Source: CAD feature listing. Evaluate the final solid. Frame: model axes, mm. Face numbers are marked on the shaded views. A direction names the side the tool comes from. Round coordinates to 2 decimals unless told otherwise and drop trailing zeros. Write each loop counter-clockwise with the first axis right and the second up, starting at its lowest first coordinate (ties: lowest second). Pieces come first, ordered by that corner, then holes. Notation, with made-up numbers: M 23.25,-2.75 L 44.25,-2.75 A12 cw 44.25,16.25 Z; hole C -5.75,-11.5 d6. An arc over 180 degrees is marked long. Answer in a Markdown table with one row per item.
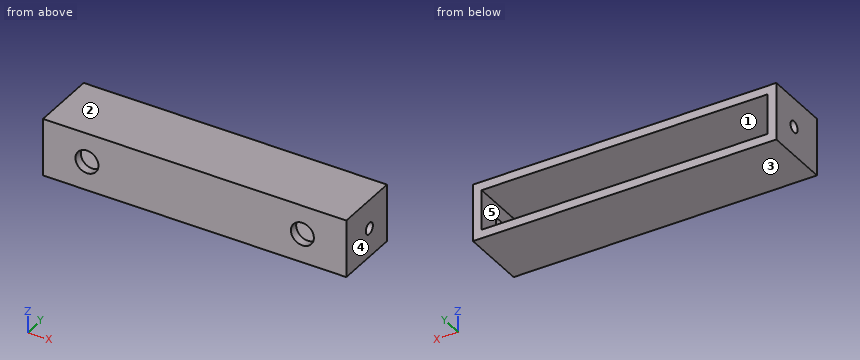
from build123d import *

# Parameters (mm, degrees)
SKETCH_1_W          = 105.6
SKETCH_1_H          = 20
SKETCH_1_R          = 4
EXTRUDE_1_DEPTH     = 3
SKETCH_10_W         = 105.6
SKETCH_10_H         = 20
SKETCH_10_W_2       = 99.6
SKETCH_10_H_2       = 14
EXTRUDE_2_DEPTH     = 20
SKETCH_11_R         = 2
CUT_EXTRUDE_1_DEPTH = 110


with BuildPart() as part:
    # 草图1 → 凸台-拉伸1 (new body)
    with BuildSketch(Plane(origin=(0, 0, 0), x_dir=(1, 0, 0), z_dir=(0, 1, 0))):
        Rectangle(SKETCH_1_W, SKETCH_1_H)
        with Locations((-37.5, 0)):
            Circle(SKETCH_1_R, mode=Mode.SUBTRACT)
        with Locations((37.5, 0)):
            Circle(SKETCH_1_R, mode=Mode.SUBTRACT)
    extrude(amount=EXTRUDE_1_DEPTH)

    # 草图10 → 凸台-拉伸2 (add)
    with BuildSketch(Plane(origin=(0, 3, 0), x_dir=(1, 0, 0), z_dir=(0, 1, 0))):
        Rectangle(SKETCH_10_W, SKETCH_10_H)
        Rectangle(SKETCH_10_W_2, SKETCH_10_H_2, mode=Mode.SUBTRACT)
    extrude(amount=EXTRUDE_2_DEPTH)

    # 草图11 → 切除-拉伸1 (cut)
    with BuildSketch(Plane.ZY.offset(52.8)):
        with Locations((0, 13)):
            Circle(SKETCH_11_R)
    extrude(amount=-CUT_EXTRUDE_1_DEPTH, mode=Mode.SUBTRACT)


solid = part.part
Q1. Section A-A (x = 37.5). Return loops of the section in (y, z), and give its area (3 significant figures).
Solutions:
| item | result |
|---|---|
| outline | M 0,-10 L 23,-10 L 23,-7 L 3,-7 L 3,-4 L 0,-4 Z; M 0,4 L 3,4 L 3,7 L 23,7 L 23,10 L 0,10 Z |
| area | 156 mm2 |
Q2. Contact query for flat-ended pins moving along their axis: pin 1 Ø9 at (x, z) = (37.5, 0) entering from +Y; pin 2 Ø5 at (x, z) = (-37.5, 0) entering from -Y. Output: stop coordinate, or through.
Solutions:
| item | result |
|---|---|
| pin 1 | stops at y = 3 |
| pin 2 | passes through |
Q3. Access query for the marked faces 1 and 2. Directions: +Z, -Z, +X, -X, +Y, -Y. A direction counts if a zero-diameter tool reaches every point of the face in a straight line with its end or side. Return the directions, or none.
Solutions:
| item | result |
|---|---|
| face 1 | +Y |
| face 2 | +Z, +X, -X, +Y, -Y |
Q4. Section D-D (x = -18). Return loops of the section in (y, z), and give its area (3 significant figures).
Solutions:
| item | result |
|---|---|
| outline | M 0,-10 L 23,-10 L 23,-7 L 3,-7 L 3,7 L 23,7 L 23,10 L 0,10 Z |
| area | 180 mm2 |
Q5. Section B-B (z = 0). Return loops of the section in (x, y), and give its area (3 significant figures).
Solutions:
| item | result |
|---|---|
| outline | M -52.8,0 L -41.5,0 L -41.5,3 L -49.8,3 L -49.8,11 L -52.8,11 Z; M -52.8,15 L -49.8,15 L -49.8,23 L -52.8,23 Z; M -33.5,0 L 33.5,0 L 33.5,3 L -33.5,3 Z; M 41.5,0 L 52.8,0 L 52.8,11 L 49.8,11 L 49.8,3 L 41.5,3 Z; M 49.8,15 L 52.8,15 L 52.8,23 L 49.8,23 Z |
| area | 365 mm2 |
Q6. Pull-direction query (Z, two-part tool) for the marked faces 3, 4 and 5; classes: pulls with the +Z half, pulls with the -Z half, needs draft (parallel to the pull), parting line crosses it, or undercut.
Solutions:
| item | result |
|---|---|
| face 3 | pulls with the -Z half |
| face 4 | needs draft |
| face 5 | undercut |
Q7. Section C-C (y = 13). Return loops of the section in (x, z).
Solutions:
| item | result |
|---|---|
| outline | M -52.8,-10 L 52.8,-10 L 52.8,-2 L 49.8,-2 L 49.8,-7 L -49.8,-7 L -49.8,-2 L -52.8,-2 Z; M -52.8,2 L -49.8,2 L -49.8,7 L 49.8,7 L 49.8,2 L 52.8,2 L 52.8,10 L -52.8,10 Z |
Q8. Material intervals for probe 1 along X at (y, z) = (1.85, 0); probe 2 along Z at (x, y) = (-24, 12); probe 3 along Z at (x, y) = (37.5, 2), sorted ascending.
Solutions:
| item | result |
|---|---|
| probe 1 | x = -52.8 to -41.5, -33.5 to 33.5, 41.5 to 52.8 |
| probe 2 | z = -10 to -7, 7 to 10 |
| probe 3 | z = -10 to -4, 4 to 10 |
